Can you work these out from the model? Positions are in its coordinate system, mm. A direction names the side the tool comes from. Round coordinates to 2 decimals unless told otherwise and drop trailing zeros. Write each loop counter-clockwise with the first axis right and the second up, starting at its lowest first coordinate (ties: lowest second). Pieces come first, ordered by that corner, then holes. Notation, with made-up numbers: M 8,34 L 55,34 A27 ccw 55,55 Z; hole C -6,33 d7. An arc over 180 degrees is marked long. Answer as a JSON object with one key per item and string values. Group by question number.
1) I'm going to push flat-ended pins straight in: pin 1 Ø5 at (y, z) = (6, 2.5) entering from -X; pin 2 Ø1.2 at (x, y) = (-14, 9) entering from -Z; pin 3 Ø0.7 at (x, z) = (17.5, -1) entering from -Y; pin 4 Ø5 at (x, y) = (-12.5, 2) entering from -Z. Where does each tip first touch, or does it pass through?
2) Suppose I cut it at D-D, the plane x = 21. Write out the boundary of the cut face in (y, z).
3) Suppose I cut it at C-C, the plane z = 3.75. Write out the boundary of the cut face in (x, y).
4) On a 3-axis mill with a long thin cutter (end or side, diameter ignored), from which of +Z, -Z, +X, -X, +Y, -Y can I reach the whole of each face in a straight line? I mean faces 5 (the flat face through (10.696, 2, -1)), 6 (the flat face through (-6, 0.919, -1)), 7 (the flat face through (-17, 1, 7.938)), 8 (the flat face through (-14, 9.555, -1)). Say none if no direction works.
5) If we mould it in two halves opening along X, with no side actions, what happens to faces 1 (the cylindrical face through (27.3, 10, 0.8)), 2 (the flat face through (-16, -8.606, -1)), 3 (the flat face through (26.571, 0, 3)), 4 (the flat face through (-4, -2.256, 6))? For each: +X half, -X half, draft (parallel to the pull), parting line (faces both ways), or undercut.
6) Suppose I cut it at A-A, the plane x = 13. Write out the boundary of the cut face in (y, z), and give its area (3 significant figures).
7) Suppose I cut it at B-B, the plane z = 0.5. Write out the boundary of the cut face in (x, y) (1 decimal).
8) Please list where these lines run through material, in increasing order: L1, parallel to X at y = -5.5, z = -1.5; L2, parallel to Y at x = -8.5, z = 3; L3, parallel to X at y = -0.75, z = 5.75. Write a range as [from, to].
from build123d import *

# Parameters (mm, degrees)
F0_W      = 50.8
F0_H      = 21.336
F1_DEPTH  = 1.5875
F2_R      = 1.5875
F3_DEPTH  = 3.175
F5_DEPTH  = 2.38125
F6_W      = 1.5875
F6_H      = 2.38125
F6_W_2    = 5.55625
F6_H_2    = 3.96875
F6_W_3    = 2.38125
F6_H_3    = 3.175
F6_W_4    = 6.35
F6_H_4    = 4.7625
F7_DEPTH  = 1.5875
F8_SIZE   = 0.254
F9_W      = 5.55625
F9_H      = 7.14375
F10_DEPTH = 2.38125
F11_SIZE  = 0.762
F12_SIZE  = 0.254
F13_R     = 5.953125
F14_DEPTH = 9.525
F15_R     = 1.190625
F16_DEPTH = 3.175
F17_W     = 14.2875
F17_H     = 7.14375
F18_DEPTH = 8.73125
F20_DEPTH = 15.24
F22_DEPTH = 11.90625
F23_W     = 3.175
F23_H     = 5.55625
F24_DEPTH = 3.175
F25_W     = 1.5875
F25_H     = 3.175
F26_DEPTH = 1.5875
F27_R     = 0.254
F28_R     = 0.508
F29_W     = 7.9375
F29_H     = 3.175
F30_DEPTH = 3.96875
F31_SIZE  = 0.762


# Not quite as in the source:
# - a length typed as a fraction of an inch, garbled in the dataset ("3 / 203.2 mm" for 3/8 in), is restored


with BuildPart() as f1:
    # F0 (on Top) → F1 (new body)
    with BuildSketch(Plane.XY):
        with Locations((2.7589667588, 1.2681204271)):
            Rectangle(F0_W, F0_H)
    extrude(amount=F1_DEPTH)

    # F2 (on face) → F3 (cut)
    with BuildSketch(Plane.XY.offset(1.5875)):
        with Locations((25.7777167588, -7.0186295729)):
            Circle(F2_R)
        with Locations((25.7777167588, 9.5548704271)):
            Circle(F2_R)
        with Locations((-20.2597832412, 9.5548704271)):
            Circle(F2_R)
        with Locations((-20.2597832412, -7.0186295729)):
            Circle(F2_R)
    extrude(amount=-F3_DEPTH, mode=Mode.SUBTRACT)

    # F4 (on face) → F5 (join)
    with BuildSketch(Plane(origin=(0, 0, 0), x_dir=(1, 0, 0), z_dir=(0, 0, -1))):
        with BuildLine():
            ThreePointArc((-5.1785332412, 6.2248795729), (-5.9722832412, 5.4311295706), (-5.1785332365, 4.6373795729))
            ThreePointArc((-5.1785332365, 4.6373795729), (-4.6172672319, 4.869863567), (-4.3847832412, 5.4311295729))
            ThreePointArc((-4.3847832412, 5.4311295729), (-4.6172672336, 5.9923955805), (-5.1785332412, 6.2248795729))
        make_face()
        with BuildLine():
            ThreePointArc((-2.0035332412, 6.2248795729), (-2.7972832412, 5.4311295729), (-2.0035332412, 4.6373795729))
            ThreePointArc((-2.0035332412, 4.6373795729), (-1.4422672336, 4.8698635653), (-1.2097832412, 5.4311295729))
            ThreePointArc((-1.2097832412, 5.4311295729), (-1.4422672336, 5.9923955805), (-2.0035332412, 6.2248795729))
        make_face()
        with BuildLine():
            ThreePointArc((1.1714667642, 6.2248795729), (0.3777167588, 5.4311295756), (1.1714667588, 4.6373795729))
            ThreePointArc((1.1714667588, 4.6373795729), (1.7327327664, 4.8698635653), (1.9652167588, 5.4311295729))
            ThreePointArc((1.9652167588, 5.4311295729), (1.7327327683, 5.9923955786), (1.1714667642, 6.2248795729))
        make_face()
        with BuildLine():
            ThreePointArc((-7.5597832412, -7.1736204271), (-7.7922672336, -6.6123544195), (-8.3535332412, -6.3798704271))
            ThreePointArc((-8.3535332412, -6.3798704271), (-9.1472832412, -7.1736204294), (-8.3535332365, -7.9673704271))
            ThreePointArc((-8.3535332365, -7.9673704271), (-7.7922672319, -7.734886433), (-7.5597832412, -7.1736204271))
        make_face()
        with BuildLine():
            ThreePointArc((-4.3085832412, -7.1736204271), (-4.5410672336, -6.6123544195), (-5.1023332412, -6.3798704271))
            ThreePointArc((-5.1023332412, -6.3798704271), (-5.8960832412, -7.1736204294), (-5.1023332365, -7.9673704271))
            ThreePointArc((-5.1023332365, -7.9673704271), (-4.5410672319, -7.734886433), (-4.3085832412, -7.1736204271))
        make_face()
        with BuildLine():
            ThreePointArc((-1.0573832412, -7.1736204271), (-1.2898672336, -6.6123544195), (-1.8511332412, -6.3798704271))
            ThreePointArc((-1.8511332412, -6.3798704271), (-2.6448832412, -7.173620426), (-1.8511332433, -7.9673704271))
            ThreePointArc((-1.8511332433, -7.9673704271), (-1.2898672344, -7.7348864354), (-1.0573832412, -7.1736204271))
        make_face()
        with BuildLine():
            ThreePointArc((2.1938167588, -7.1736204271), (1.9613327682, -6.6123544213), (1.4000667639, -6.3798704271))
            ThreePointArc((1.4000667639, -6.3798704271), (0.6063167588, -7.1736204215), (1.4000667527, -7.9673704271))
            ThreePointArc((1.4000667527, -7.9673704271), (1.9613327642, -7.7348864368), (2.1938167588, -7.1736204271))
        make_face()
        with BuildLine():
            ThreePointArc((-8.3535332412, 6.2248795729), (-9.1472832412, 5.4311295729), (-8.3535332412, 4.6373795729))
            ThreePointArc((-8.3535332412, 4.6373795729), (-7.7922672336, 4.8698635653), (-7.5597832412, 5.4311295729))
            ThreePointArc((-7.5597832412, 5.4311295729), (-7.7922672336, 5.9923955805), (-8.3535332412, 6.2248795729))
        make_face()
    extrude(amount=F5_DEPTH)

    # F6 (on face) → F7 (join)
    with BuildSketch(Plane(origin=(0, 0, 0), x_dir=(1, 0, 0), z_dir=(0, 0, -1))):
        with Locations((-15.4972832412, 7.4155045729)):
            Rectangle(F6_W, F6_H)
        with Locations((-15.4972832412, 4.2405045729)):
            Rectangle(F6_W, F6_H)
        with Locations((-13.9097832412, -8.3642454271)):
            Rectangle(F6_W, F6_H)
        with Locations((-6.3691582412, 1.0655045729)):
            Rectangle(F6_W_2, F6_H_2)
        with Locations((0.7745917588, -0.1251204271)):
            Rectangle(F6_W_3, F6_H_3)
        with Locations((18.6339667588, 1.4623795729)):
            Rectangle(F6_W_4, F6_H_4)
        with Locations((18.2370917588, -4.7923704271)):
            Rectangle(F6_W_3, F6_H_4)
    extrude(amount=F7_DEPTH)

    # F8
    f8_edges = [f1.edges().sort_by_distance(p)[0] for p in [
        (-13.909783, 9.55487, -1.5875),
        (-13.116033, 8.364245, -1.5875),
        (-13.909783, 7.17362, -1.5875),
        (-14.703533, 8.364245, -1.5875),
        (-15.497283, -5.43113, -1.5875),
        (-16.291033, -4.240505, -1.5875),
        (-15.497283, -3.04988, -1.5875),
        (-14.703533, -4.240505, -1.5875),
        (-15.497283, -8.60613, -1.5875),
        (-16.291033, -7.415505, -1.5875),
        (-15.497283, -6.22488, -1.5875),
        (-14.703533, -7.415505, -1.5875),
        (-3.591033, -1.065505, -1.5875),
        (-6.369158, -3.04988, -1.5875),
        (-9.147283, -1.065505, -1.5875),
        (-6.369158, 0.91887, -1.5875),
        (0.774592, 1.71262, -1.5875),
        (1.965217, 0.12512, -1.5875),
        (0.774592, -1.46238, -1.5875),
        (-0.416033, 0.12512, -1.5875),
        (18.633967, 0.91887, -1.5875),
        (21.808967, -1.46238, -1.5875),
        (18.633967, -3.84363, -1.5875),
        (15.458967, -1.46238, -1.5875),
        (19.427717, 4.79237, -1.5875),
        (18.237092, 2.41112, -1.5875),
        (17.046467, 4.79237, -1.5875),
        (18.237092, 7.17362, -1.5875),
    ]]
    chamfer(f8_edges, length=F8_SIZE)

    # F9 (on face) → F10 (join)
    with BuildSketch(Plane(origin=(0, 0, 0), x_dir=(1, 0, 0), z_dir=(0, 0, -1))):
        with Locations((7.9183417588, -2.1094954271)):
            Rectangle(F9_W, F9_H)
    extrude(amount=F10_DEPTH)

    # F11
    f11_edges = [f1.edges().sort_by_distance(p)[0] for p in [
        (10.696467, 2.109495, -2.38125),
        (5.140217, 2.109495, -2.38125),
    ]]
    chamfer(f11_edges, length=F11_SIZE)

    # F12
    f12_edges = [f1.edges().sort_by_distance(p)[0] for p in [
        (7.918342, -1.46238, -2.38125),
        (7.918342, 5.68137, -2.38125),
    ]]
    chamfer(f12_edges, length=F12_SIZE)

    # F13 (on face) → F14 (join)
    with BuildSketch(Plane.XY.offset(1.5875)):
        with Locations((-16.6879082412, 1.2204954271)):
            Circle(F13_R)
    extrude(amount=F14_DEPTH)

    # F15 (on face) → F16 (cut)
    with BuildSketch(Plane.XY.offset(11.1125)):
        with Locations((-16.6879082412, 1.2204954271)):
            Circle(F15_R)
    extrude(amount=-F16_DEPTH, mode=Mode.SUBTRACT)

    # F17 (on face) → F18 (join)
    with BuildSketch(Plane.XY.offset(1.5875)):
        with Locations((-3.5910332412, 8.3642454271)):
            Rectangle(F17_W, F17_H)
        with Locations((-3.5910332412, -5.8280045729)):
            Rectangle(F17_W, F17_H)
    extrude(amount=F18_DEPTH)

    # F19 (on face) → F20 (cut)
    with BuildSketch(Plane.YZ.offset(3.5527167588)):
        Polygon((-12.6245096326, 12.3970924459), (-9.3998795729, 7.14375), (-7.8123795729, 10.31875), (-6.8544447422, 13.4305364035), align=None)
        Polygon((11.640425374, 13.160722746), (10.3486204271, 10.31875), (11.9361204271, 7.14375), (15.5531742786, 9.6412404954), (16.3770463069, 13.6774447247), align=None)
    extrude(amount=-F20_DEPTH, mode=Mode.SUBTRACT)

    # F21 (on face) → F22 (join)
    with BuildSketch(Plane.YZ.offset(3.5527167588)):
        with BuildLine():
            ThreePointArc((1.9973354259, 1.6797255876), (3.8268101171, 2.8522266244), (4.5383704271, 4.905375))
            ThreePointArc((4.5383704271, 4.905375), (-0.8326529485, 7.51168969), (0.4436554283, 1.6797255876))
            Line((0.4436554283, 1.6797255876), (1.9973354259, 1.6797255876))
        make_face()
        with BuildLine():
            Line((1.9973354259, 1.6797255876), (0.4436554283, 1.6797255876))
            ThreePointArc((0.4436554283, 1.6797255876), (1.2204954271, 1.5875), (1.9973354259, 1.6797255876))
        make_face()
        with BuildLine():
            ThreePointArc((1.9973354259, 1.6797255876), (1.2204954271, 1.5875), (0.4436554283, 1.6797255876))
            Line((0.4436554283, 1.6797255876), (0.4436554283, 1.5345554566))
            Line((0.4436554283, 1.5345554566), (1.9973354259, 1.5345554566))
            Line((1.9973354259, 1.5345554566), (1.9973354259, 1.6797255876))
        make_face()
    extrude(amount=-F22_DEPTH)

    # F23 (on face) → F24 (join)
    with BuildSketch(Plane.XY.offset(1.5875)):
        with Locations((24.9839667588, 0.5219954271)):
            Rectangle(F23_W, F23_H)
    extrude(amount=F24_DEPTH)

    # F25 (on face) → F26 (join)
    with BuildSketch(Plane.XY.offset(4.7625)):
        with Locations((24.9839667588, 0.5219954271)):
            Rectangle(F25_W, F25_H)
    extrude(amount=F26_DEPTH)

    # F27
    f27_edges = [f1.edges().sort_by_distance(p)[0] for p in [
        (25.777717, -1.065505, 5.55625),
        (24.190217, -1.065505, 5.55625),
        (24.190217, 2.109495, 5.55625),
        (25.777717, 2.109495, 5.55625),
    ]]
    fillet(f27_edges, radius=F27_R)

    # F28
    f28_edges = [f1.edges().sort_by_distance(p)[0] for p in [
        (26.571467, 3.30012, 3.175),
        (23.396467, 3.30012, 3.175),
        (26.571467, -2.25613, 3.175),
        (23.396467, -2.25613, 3.175),
    ]]
    fillet(f28_edges, radius=F28_R)

    # F29 (on face) → F30 (join)
    with BuildSketch(Plane.XY.offset(1.5875)):
        with Locations((9.9027167588, -7.8123795729)):
            Rectangle(F29_W, F29_H)
    extrude(amount=F30_DEPTH)

    # F31
    f31_edges = [f1.edges().sort_by_distance(p)[0] for p in [
        (9.902717, -9.39988, 5.55625),
    ]]
    chamfer(f31_edges, length=F31_SIZE)


solid = f1.part
Results:
{
 "1": {"pin 1": "x = -22.64", "pin 2": "z = -1.59", "pin 3": "y = -3.84", "pin 4": "z = 0"},
 "2": {"outline": "M -9.4,0 L -3.84,0 L -3.84,-1.33 L -3.59,-1.59 L 0.66,-1.59 L 0.92,-1.33 L 0.92,0 L 11.94,0 L 11.94,1.59 L -9.4,1.59 Z"},
 "3": {"outline": "C -16.69,1.22 d11.91; M -10.73,-9.4 L 3.55,-9.4 L 3.55,-2.26 L -10.73,-2.26 Z; M -10.73,4.79 L 3.55,4.79 L 3.55,11.94 L -10.73,11.94 Z; M -8.35,-1.89 L 3.55,-1.89 L 3.55,4.33 L -8.35,4.33 Z; M 5.93,-9.4 L 13.87,-9.4 L 13.87,-6.22 L 5.93,-6.22 Z; M 23.4,-1.75 A0.51 ccw 23.9,-2.26 L 26.06,-2.26 A0.51 ccw 26.57,-1.75 L 26.57,2.79 A0.51 ccw 26.06,3.3 L 23.9,3.3 A0.51 ccw 23.4,2.79 Z"},
 "4": {"face 5": "-Z, +Y, -Y", "face 6": "-Z, -X", "face 7": "+Z", "face 8": "-Z, +X, -X, +Y"},
 "5": {"face 1": "undercut", "face 2": "draft", "face 3": "+X half", "face 4": "undercut"},
 "6": {"outline": "M -9.4,0 L 11.94,0 L 11.94,1.59 L -6.22,1.59 L -6.22,5.56 L -8.64,5.56 L -9.4,4.79 Z", "area": "46.2 mm^2"},
 "7": {"outline": "M -22.6,-9.4 L 28.2,-9.4 L 28.2,11.9 L -22.6,11.9 Z; hole C -20.3,-7 d3.2; hole C -20.3,9.6 d3.2; hole C 25.8,-7 d3.2; hole C 25.8,9.6 d3.2"},
 "8": {"L1": "[-9.14, -7.56], [-5.97, -4.39], [-2.79, -1.21], [0.38, 1.96]", "L2": "[-9.4, -2.26], [4.79, 11.94]", "L3": "[-22.31, -11.07], [-8.35, 3.55], [24.19, 25.78]"}
}
